The listing builds one solid part. Answer for the finished solid, in the listing's coordinates (mm). Face numbers are marked on the shaded views. Give positions to 0.01 mm unless a question says otherwise; leave off trailing zeros. Write each loop counter-clockwise with the first axis right and the second up, starting at its lowest first coordinate (ties: lowest second). Pieces come first, ordered by that corner, then holes. Notation, with made-up numbers: (76.5, 14.5) -> (128.5, 14.5) arc R6 ccw to (128.5, 19.5) -> close; hole circle Ø3 at (-20, -25.5). An arc over 180 degrees is marked (long way). One line per question, with ' | ' between items.
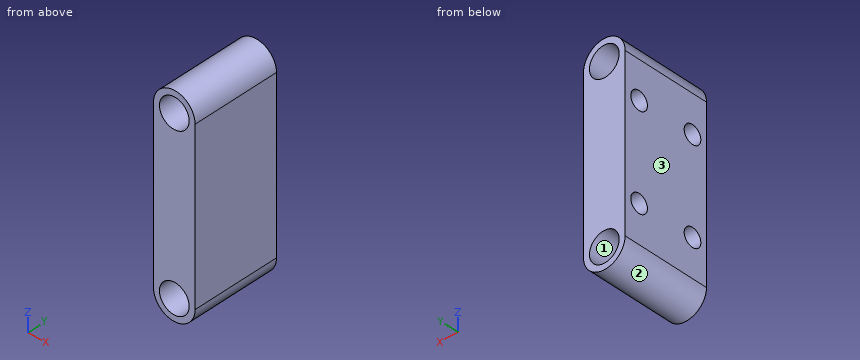
from build123d import *

# Parameters (mm, degrees)
SKETCH2_R           = 3.175
BOSS_EXTRUDE1_DEPTH = 9.525
SKETCH3_R           = 1.95
CUT_EXTRUDE1_DEPTH  = 5.8


with BuildPart() as part:
    # Sketch2 → Boss-Extrude1 (new body, symmetric)
    with BuildSketch(Plane(origin=(0, 0, 0), x_dir=(1, 0, 0), z_dir=(0, 1, 0))):
        with BuildLine():
            Line((13.515512242, 17.960512242), (13.515512242, -17.960512242))
            ThreePointArc((13.515512242, -17.960512242), (17.960512242, -22.405512242), (22.405512242, -17.960512242))
            Line((22.405512242, -17.960512242), (22.405512242, 17.960512242))
            ThreePointArc((22.405512242, 17.960512242), (17.960512242, 22.405512242), (13.515512242, 17.960512242))
        make_face()
        with Locations((17.960512242, -17.960512242)):
            Circle(SKETCH2_R, mode=Mode.SUBTRACT)
        with Locations((17.960512242, 17.960512242)):
            Circle(SKETCH2_R, mode=Mode.SUBTRACT)
    extrude(amount=BOSS_EXTRUDE1_DEPTH, both=True)

    # Sketch3 → Cut-Extrude1 (cut)
    with BuildSketch(Plane.ZY.offset(-13.515512242)):
        with Locations((-9.97, 6.25)):
            Circle(SKETCH3_R)
        with Locations((9.97, 6.25)):
            Circle(SKETCH3_R)
        with Locations((9.97, -6.25)):
            Circle(SKETCH3_R)
        with Locations((-9.97, -6.25)):
            Circle(SKETCH3_R)
    extrude(amount=-CUT_EXTRUDE1_DEPTH, mode=Mode.SUBTRACT)


solid = part.part
Item 1: Flat-ended cylindrical pins translate along their axes: pin 1 (1.2 mm diameter, centred on y = -5.5, z = -10.5, fed in from -X); pin 2 (4.5 mm diameter, centred on y = -6.25, z = 9.97, fed in from -X); pin 3 (5 mm diameter, centred on x = 17.96, z = 17.96, fed in from -Y); pin 4 (1 mm diameter, centred on x = 20.5, y = -7.5, fed in from -Z). Find the tip coordinate at first contact, or state that the pin passes through.
Answers below:
pin 1: x = 19.32 | pin 2: x = 13.52 | pin 3: through | pin 4: z = -21.91
Item 2: Find section B-B (y = 1.25). Write down the section's boundary in (x, z) (3 decimals).
Answers below:
outline: (13.516, -17.961) arc R4.445 ccw to (22.406, -17.961) -> (22.406, 17.961) arc R4.445 ccw to (13.516, 17.961) -> close; hole circle Ø6.35 at (17.961, -17.961); hole circle Ø6.35 at (17.961, 17.961)
Item 3: Determine the mould class of the marked faces 1, 2 and 3 for opening direction Z: pulls with the +Z half, pulls with the -Z half, needs draft (parallel to the pull), parting line crosses it, or undercut.
Answers below:
face 1: undercut | face 2: pulls with the -Z half | face 3: needs draft
Item 4: Find section A-A (x = 17.25). Write down the section's boundary in (y, z) (3 decimals).
Answers below:
outline: (-9.525, -22.348) -> (9.525, -22.348) -> (9.525, -21.055) -> (-9.525, -21.055) -> close; (-9.525, -14.866) -> (9.525, -14.866) -> (9.525, 14.866) -> (-9.525, 14.866) -> close; (-9.525, 21.055) -> (9.525, 21.055) -> (9.525, 22.348) -> (-9.525, 22.348) -> close; hole circle Ø3.9 at (-6.25, -9.97); hole circle Ø3.9 at (-6.25, 9.97); hole circle Ø3.9 at (6.25, -9.97); hole circle Ø3.9 at (6.25, 9.97)
Item 5: Find section C-C (z = 9.97). Write down the section's boundary in (x, y) (3 decimals).
Answers below:
outline: (13.516, -9.525) -> (22.406, -9.525) -> (22.406, 9.525) -> (13.516, 9.525) -> (13.516, 8.2) -> (19.316, 8.2) -> (19.316, 4.3) -> (13.516, 4.3) -> (13.516, -4.3) -> (19.316, -4.3) -> (19.316, -8.2) -> (13.516, -8.2) -> close
Item 6: Find section D-D (z = -19.5). Write down the section's boundary in (x, y) (3 decimals).
Answers below:
outline: (13.791, -9.525) -> (15.184, -9.525) -> (15.184, 9.525) -> (13.791, 9.525) -> close; (20.737, -9.525) -> (22.13, -9.525) -> (22.13, 9.525) -> (20.737, 9.525) -> close
Item 7: Consider line 1 (Y direction, x = 16.2, z = 9.97) (3 decimals); line 2 (Z direction, x = 15.75, y = -4.5); line 3 (Z direction, x = 18, y = 5). Determine where each line is inside the solid, lowest interval first. Write a range as [from, to].
Answers below:
line 1: [-9.525, -8.2], [-4.3, 4.3], [8.2, 9.525] | line 2: [-21.82, -20.24], [-15.68, -10.83], [-9.11, 9.11], [10.83, 15.68], [20.24, 21.82] | line 3: [-22.41, -21.14], [-14.79, -11.47], [-8.47, 8.47], [11.47, 14.79], [21.14, 22.41]
